Read the model definition and answer for the solid it produces. Units are mm, in the model's axes. A direction names the side the tool comes from. Coordinates: 2 decimals unless noted, no trailing zeros. Order: outer loops, then holes, each group sorted by start corner. A loop starts at its lowest first (then second) coordinate and runs counter-clockwise, first axis right, second up. Notation, with made-up numbers: (-4, 34) -> (50, 34) arc R22 cw to (50, 59) -> close; hole circle Ø2 at (83.5, 7). An arc over 180 degrees is marked (long way). Use CSV: the item, a comma, the result in double quotes.
```python
from build123d import *

# Parameters (mm, degrees)
BOSS_EXTRUDE1_DEPTH      = 10
BOSS_EXTRUDE2_DEPTH      = 42
BOSS_EXTRUDE2_DEPTH_BACK = 10
BOSS_EXTRUDE3_DEPTH      = 10
SKETCH3_R                = 20.035
CUT_EXTRUDE2_DEPTH       = 10
FILLET1_R                = 12
SKETCH9_W                = 7.5
SKETCH9_H                = 4
BOSS_EXTRUDE5_DEPTH      = 4
FILLET4_R                = 1.95
FILLET5_R                = 3
FILLET6_R                = 3
SKETCH10_R               = 3
CUT_EXTRUDE3_DEPTH       = 10


with BuildPart() as part:
    # Sketch1 → Boss-Extrude1 (new body)
    with BuildSketch(Plane(origin=(0, 0, 0), x_dir=(1, 0, 0), z_dir=(0, 1, 0))):
        Polygon((0, 0), (-43.5, 0), (-43.5, -68), (23, -68), (23, 0), align=None)
    extrude(amount=BOSS_EXTRUDE1_DEPTH)

    # Sketch2 → Boss-Extrude2 (add, two sides)
    with BuildSketch(Plane.XZ) as boss_extrude2_sk:
        Polygon((-43.5, 68), (-43.5, 62), (23, 62), (23, 68), (23, 75), (-43.5, 75), align=None)
    extrude(amount=BOSS_EXTRUDE2_DEPTH)
    extrude(boss_extrude2_sk.sketch, amount=-BOSS_EXTRUDE2_DEPTH_BACK)

    # Sketch4 → Boss-Extrude3 (add)
    with BuildSketch(Plane.XZ):
        Polygon((-43.5, 62), (-36, 62), (-36, 7.5), (15.5, 7.5), (15.5, 62), (23, 62), (23, 0), (-43.5, 0), align=None)
    extrude(amount=BOSS_EXTRUDE3_DEPTH)

    # Sketch3 → Cut-Extrude2 (cut)
    with BuildSketch(Plane(origin=(0, 0, 0), x_dir=(-1, 0, 0), z_dir=(0, 0, -1))):
        with Locations((16, -22)):
            Circle(SKETCH3_R)
    extrude(amount=-CUT_EXTRUDE2_DEPTH, mode=Mode.SUBTRACT)

    # Fillet1
    fillet1_edges = [part.edges().sort_by_distance(p)[0] for p in [
        (19.25, -10, 62),
        (-39.75, -10, 62),
    ]]
    fillet(fillet1_edges, radius=FILLET1_R)

    # Sketch9 → Boss-Extrude5 (add)
    with BuildSketch(Plane.XZ.offset(10)):
        with Locations((-39.75, 27)):
            Rectangle(SKETCH9_W, SKETCH9_H)
        with Locations((19.25, 27)):
            Rectangle(SKETCH9_W, SKETCH9_H)
    extrude(amount=BOSS_EXTRUDE5_DEPTH)

    # Fillet4
    fillet4_edges = [part.edges().sort_by_distance(p)[0] for p in [
        (-10.25, -42, 62),
    ]]
    fillet(fillet4_edges, radius=FILLET4_R)

    # Fillet5
    fillet5_edges = [part.edges().sort_by_distance(p)[0] for p in [
        (23, 0, 0),
        (-43.5, 0, 0),
    ]]
    fillet(fillet5_edges, radius=FILLET5_R)

    # Fillet6
    fillet6_edges = [part.edges().sort_by_distance(p)[0] for p in [
        (-10.25, 10, 0),
        (-43.5, 10, 39),
        (-42.621320344, 10, 0.878679656),
        (22.121320344, 10, 0.878679656),
        (23, 10, 39),
        (-10.25, 10, 75),
    ]]
    fillet(fillet6_edges, radius=FILLET6_R)

    # Sketch10 → Cut-Extrude3 (cut)
    with BuildSketch(Plane.XZ.offset(42)):
        with Locations((-28.5, 68)):
            Circle(SKETCH10_R)
        with Locations((5.5, 68)):
            Circle(SKETCH10_R)
    extrude(amount=-CUT_EXTRUDE3_DEPTH, mode=Mode.SUBTRACT)


solid = part.part
```
Item 1: Each of these flat-tipped pins is pushed along its axis until it touches: P1, Ø10, axis at x = -7, y = -24, coming from the -Z side; P2, Ø6, axis at x = 14.5, z = 26, coming from the -Y side; P3, Ø7, axis at x = -28.5, z = 68, coming from the -Y side; P4, Ø6, axis at x = 20.5, z = 40, coming from the -Y side. Where does it stop, or does it pass through?
Return value:
P1,"stops at z = 62"
P2,"stops at y = -14"
P3,"stops at y = -42"
P4,"stops at y = -10"
Item 2: Find section B-B, the plane z = 68. Give the vertices of the cut face in (x, y), then the cut area to 3 significant figures.
Return value:
outline,"(-43.5, -42) -> (-31.5, -42) -> (-31.5, -32) -> (-25.5, -32) -> (-25.5, -42) -> (2.5, -42) -> (2.5, -32) -> (8.5, -32) -> (8.5, -42) -> (23, -42) -> (23, 7) arc R3 ccw to (20, 10) -> (-40.5, 10) arc R3 ccw to (-43.5, 7) -> close"
area,"3,330 mm^2"
Item 3: Find section A-A, the plane x = 17. Give the vertices of the cut face in (y, z), then the cut area to 3 significant figures.
Return value:
outline,"(-42, 63.95) arc R1.95 ccw to (-40.05, 62) -> (-22, 62) arc R12 cw to (-10, 50) -> (-10, 29) -> (-14, 29) -> (-14, 25) -> (-10, 25) -> (-10, 0) -> (7, 0) arc R3 ccw to (10, 3) -> (10, 72) arc R3 ccw to (7, 75) -> (-42, 75) -> close"
area,"1,960 mm^2"
Item 4: Find section D-D, the plane x = 5.5. Give the vertices of the cut face in (y, z).
Return value:
outline,"(-42, 63.95) arc R1.95 ccw to (-40.05, 62) -> (0, 62) -> (0, 7.5) -> (-10, 7.5) -> (-10, 0) -> (7, 0) arc R3 ccw to (10, 3) -> (10, 72) arc R3 ccw to (7, 75) -> (-42, 75) -> (-42, 71) -> (-32, 71) -> (-32, 65) -> (-42, 65) -> close"
Item 5: Straight lines are drawn through the part: line 1 along Z through (x, y) = (-28.5, -38); line 2 along X through (y, z) = (-8, 42); line 3 along Z through (x, y) = (-2.5, -5). For each, find the intervals that lie inside material, in ascending order.
Return value:
line 1,"z = 62 to 65, 71 to 75"
line 2,"x = -43.5 to -36, 15.5 to 23"
line 3,"z = 0 to 7.5, 62 to 75"
Item 6: Find section C-C, the plane y = -30.5. Give the vertices of the cut face in (x, z), then the cut area to 4 significant figures.
Return value:
outline,"(-43.5, 62) -> (23, 62) -> (23, 75) -> (-43.5, 75) -> close"
area,"864.5 mm^2"
Item 7: A tool of negligible diameter and unlimited length cuts with its end or side. For faces 1 (the flat face through (23, -6, 46)), 2 (the cylindrical face through (19.3, -13.61, 58.58)), 3 (the flat face through (-11, -20, 62)), from which of +Z, -Z, +X, -X, +Y, -Y can it reach the whole face along a straight path? Write none if from no direction.
Return value:
face 1,"+Z, -Z, +X, +Y, -Y"
face 2,"+X, -X, -Y"
face 3,"-Y"
Item 8: The mould has two halves that part along Z. Classify faces 4 (the cylindrical face through (-10.72, 9.14, 74.1)), 5 (the flat face through (19, -10, 40)), 6 (the flat face through (17, -10, 10)), 7 (the flat face through (-40, -10, 40)): +Z half, -Z half, draft (parallel to the pull), parting line (faces both ways), or undercut.
Return value:
face 4,"+Z half"
face 5,"undercut"
face 6,"draft"
face 7,"undercut"
